from build123d import *

# Parameters (mm, degrees)
SKETCH1_W           = 15
SKETCH1_H           = 15
SKETCH1_W_2         = 12.5
SKETCH1_H_2         = 12.5
BOSS_EXTRUDE1_DEPTH = 238.95
SKETCH2_R           = 1.95
CUT_EXTRUDE1_DEPTH  = 240.537789294
SKETCH5_R           = 3.75
SKETCH5_R_2         = 2
CUT_EXTRUDE6_DEPTH  = 5


with BuildPart() as part:
    # Sketch1 → Boss-Extrude1 (new body)
    with BuildSketch(Plane(origin=(0, 0, 0), x_dir=(0, 0, -1), z_dir=(1, 0, 0))):
        Rectangle(SKETCH1_W, SKETCH1_H)
        Rectangle(SKETCH1_W_2, SKETCH1_H_2, mode=Mode.SUBTRACT)
    extrude(amount=BOSS_EXTRUDE1_DEPTH)

    # Sketch2 → Cut-Extrude1 (cut, through all)
    with BuildSketch(Plane(origin=(0, 0, -7.5), x_dir=(-1, 0, 0), z_dir=(0, 0, -1))):
        with Locations(Location((-12.000000001, 0, 0), (0, 0, 90))):
            Circle(SKETCH2_R)
        with Locations(Location((-32.000000001, 0, 0), (0, 0, 90))):
            Circle(SKETCH2_R)
    extrude(amount=-CUT_EXTRUDE1_DEPTH, mode=Mode.SUBTRACT)

    # Sketch5 → Cut-Extrude6 (cut)
    with BuildSketch(Plane.XZ.offset(7.5)):
        with Locations(Location((64.7, 0, 0), (0, 0, 270))):
            Circle(SKETCH5_R)
        with Locations(Location((228.95, 0, 0), (0, 0, 270))):
            Circle(SKETCH5_R_2)
    extrude(amount=-CUT_EXTRUDE6_DEPTH, mode=Mode.SUBTRACT)


solid = part.part
Read the model definition and answer for the solid it produces. Units are mm, in the model's axes. A direction names the side the tool comes from. Round coordinates to 2 decimals unless told otherwise and drop trailing zeros. Order: outer loops, then holes, each group sorted by start corner. A loop starts at its lowest first (then second) coordinate and runs counter-clockwise, first axis right, second up. Notation, with made-up numbers: (36, -16) - (78, -16) arc R15 cw to (78, 7) - close; hole circle Ø5 at (87.5, 71). An arc over 180 degrees is marked (long way). Use one line per item in the form item = value. Start each with the question number.
(1) Determine the mould class of faces 4 (the face through (118, 0, -6.25)), 5 (the face through (227.176, -6.884, -0.923)), 6 (the face through (0, 0, 7)), 7 (the face through (10.096, -0.423, -6.884)) for opening direction X: +X half, -X half, draft (parallel to the pull), parting line (faces both ways), or undercut.
(2) The part is cut by section C-C (x = 64.7). Give the vertices of the cut face in (y, z), then the cut area to 3 significant figures.
(3) The part is cut by section D-D (x = 32). Give the vertices of the cut face in (y, z).
(4) The part is cut by section A-A (z = 0). Give the vertices of the cut face in (x, y).
(5) The part is cut by section B-B (y = 0). Give the vertices of the cut face in (x, z), then the cut area to 3 significant figures.
(6) Find the intervals of material crossed by line 1 along X through (y, z) = (0, -6.9); line 2 along X through (y, z) = (-6.65, 0); line 3 along Z through (x, y) = (228.95, -7.1), in increasing order. Write a range as from..to.
(7) For faces 1 (the face through (118, 6.25, 0)), 2 (the face through (68.418, -6.884, 0.488)), 3 (the face through (32.59, 1.86, 6.87)), determine the directions among +Z, -Z, +X, -X, +Y, -Y from which every point of the face is accessible in a straight line to the end or side of a thin tool.
Checked values:
q1.face_4 = draft
q1.face_5 = undercut
q1.face_6 = -X half
q1.face_7 = undercut
q2.outline = (-7.5, -7.5) - (7.5, -7.5) - (7.5, 7.5) - (-7.5, 7.5) - (-7.5, 3.75) - (-6.25, 3.75) - (-6.25, 6.25) - (6.25, 6.25) - (6.25, -6.25) - (-6.25, -6.25) - (-6.25, -3.75) - (-7.5, -3.75) - close
q2.area = 59.4 mm^2
q3.outline = (-7.5, -7.5) - (-1.95, -7.5) - (-1.95, -6.25) - (-6.25, -6.25) - (-6.25, 6.25) - (-1.95, 6.25) - (-1.95, 7.5) - (-7.5, 7.5) - close; (1.95, -7.5) - (7.5, -7.5) - (7.5, 7.5) - (1.95, 7.5) - (1.95, 6.25) - (6.25, 6.25) - (6.25, -6.25) - (1.95, -6.25) - close
q4.outline = (0, -7.5) - (60.95, -7.5) - (60.95, -6.25) - (0, -6.25) - close; (0, 6.25) - (238.95, 6.25) - (238.95, 7.5) - (0, 7.5) - close; (68.45, -7.5) - (226.95, -7.5) - (226.95, -6.25) - (68.45, -6.25) - close; (230.95, -7.5) - (238.95, -7.5) - (238.95, -6.25) - (230.95, -6.25) - close
q5.outline = (0, -7.5) - (10.05, -7.5) - (10.05, -6.25) - (0, -6.25) - close; (0, 6.25) - (10.05, 6.25) - (10.05, 7.5) - (0, 7.5) - close; (13.95, -7.5) - (30.05, -7.5) - (30.05, -6.25) - (13.95, -6.25) - close; (13.95, 6.25) - (30.05, 6.25) - (30.05, 7.5) - (13.95, 7.5) - close; (33.95, -7.5) - (238.95, -7.5) - (238.95, -6.25) - (33.95, -6.25) - close; (33.95, 6.25) - (238.95, 6.25) - (238.95, 7.5) - (33.95, 7.5) - close
q5.area = 578 mm^2
q6.line_1 = 0..10.05, 13.95..30.05, 33.95..238.95
q6.line_2 = 0..60.95, 68.45..226.95, 230.95..238.95
q6.line_3 = -7.5..-2, 2..7.5
q7.face_1 = +X, -X
q7.face_2 = -Y
q7.face_3 = +Z, -Z
